The model under review builds one solid part; all positions refer to its coordinate system, in mm. A direction names the side the tool comes from. Round coordinates to 2 decimals unless told otherwise and drop trailing zeros. Order: outer loops, then holes, each group sorted by start corner. A loop starts at its lowest first (then second) coordinate and runs counter-clockwise, first axis right, second up.
1) Consider section B-B (z = -4.25). Give the boundary of the cut face in (x, y).
2) Consider section D-D (z = -24.5). Give the boundary of the cut face in (x, y).
3) Mouldability with a two-part tool opening along Z and no side actions: class faces 1 (the face through (2.521, -26.767, -5.591)), 2 (the face through (-2, -20, -8.5)), 3 (the face through (2, 0, -14)) as pulls with the +Z half, pulls with the -Z half, needs draft (parallel to the pull), parting line crosses it, or undercut.
4) Machinability: for faces 4 (the face through (1, -8, -4)), 5 (the face through (0, -20, 7)), 6 (the face through (8, -20, -44.5)), which of the approach directions +Z, -Z, +X, -X, +Y, -Y give a long, thin tool a straight path to every point of the face, cutting with its end or side? Answer none if there is none.
5) Clearance check with flat-ended pins moving along their axes: P1, Ø4, axis at y = -26.5, z = 4.5, coming from the -X side; P2, Ø11, axis at y = -30, z = -4.25, coming from the +X side; P3, Ø2, axis at y = -11, z = -5, coming from the +X side. State where each tip first meets the part, or that it passes through.
6) To check wall thickness, follow L1, parallel to Y at x = -2.55, z = -4.25; L2, parallel to Z at x = 2.7, y = -10; L3, parallel to Z at x = -0.85, y = -30. State the ranges of each line that lie inside material, in increasing order.
7) Consider section A-A (x = 6.5). Give the boundary of the cut face in (y, z), then the cut area to 3 significant figures.
from build123d import *

# Parameters (mm, degrees)
F1_DEPTH = 40
F2_R     = 1.5
F3_DEPTH = 25
F5_R     = 1
F4_R     = 3.5
F4_R_2   = 1.5
F6_DEPTH = 3
F7_R     = 0.99999


# Not quite as in the source:
# - a fillet or chamfer is up to 0.001 mm smaller than in the source, because OpenCascade refuses the exact size


with BuildPart() as f1:
    # F0 (on Front) → F1 (new body)
    with BuildSketch(Plane.XZ):
        Polygon((13, 15), (0, 15), (0, 0), (-5, 0), (-5, -8.5), (0, -8.5), (0, -48.5), (13, -48.5), (13, -42.5), (11, -42.5), (11, -44.5), (4, -44.5), (4, 11), (11, 11), (11, 9), (13, 9), align=None)
    extrude(amount=F1_DEPTH)

    # F2 (on face) → F3 (cut)
    with BuildSketch(Plane(origin=(-5, 0, 0), x_dir=(0, -1, 0), z_dir=(-1, 0, 0))):
        with Locations((10, -4.25)):
            Circle(F2_R)
        with Locations((30, -4.25)):
            Circle(F2_R)
    extrude(amount=-F3_DEPTH, mode=Mode.SUBTRACT)

    # F5
    f5_edges = [f1.edges().sort_by_distance(p)[0] for p in [
        (-5, -20, 0),
        (-5, -20, -8.5),
    ]]
    fillet(f5_edges, radius=F5_R)

    # F4 (on face) → F6 (cut)
    with BuildSketch(Plane.YZ.offset(4)):
        with Locations((-10, -4.25)):
            Circle(F4_R)
        with Locations((-10, -4.25)):
            Circle(F4_R_2, mode=Mode.SUBTRACT)
        with Locations((-30, -4.25)):
            Circle(F4_R)
        with Locations((-30, -4.25)):
            Circle(F4_R_2, mode=Mode.SUBTRACT)
    extrude(amount=-F6_DEPTH, mode=Mode.SUBTRACT)

    # F7 (radius 1 in the source; OpenCascade refuses exactly that, so slightly less here)
    f7_edges = [f1.edges().sort_by_distance(p)[0] for p in [
        (13, -20, 9),
        (11, -20, 9),
        (13, -20, 15),
        (0, -20, 15),
        (4, -20, 11),
        (0, -20, -48.5),
        (13, -20, -48.5),
        (13, -20, -42.5),
        (4, -20, -44.5),
        (11, -20, -42.5),
        (11, -20, -44.5),
        (11, -20, 11),
    ]]
    fillet(f7_edges, radius=F7_R)


solid = f1.part
Answer below:
1. outline: (-5, -40) - (4, -40) - (4, -33.5) - (1, -33.5) - (1, -31.5) - (-5, -31.5) - close; (-5, -28.5) - (1, -28.5) - (1, -26.5) - (4, -26.5) - (4, -13.5) - (1, -13.5) - (1, -11.5) - (-5, -11.5) - close; (-5, -8.5) - (1, -8.5) - (1, -6.5) - (4, -6.5) - (4, 0) - (-5, 0) - close
2. outline: (0, -40) - (4, -40) - (4, 0) - (0, 0) - close
3. face 1: undercut
3. face 2: pulls with the -Z half
3. face 3: needs draft
4. face 4: +X
4. face 5: +Z, -X, +Y, -Y
4. face 6: +Y, -Y
5. P1: stops at x = 0
5. P2: stops at x = 4
5. P3: stops at x = 1
6. L1: y = -40 to -31.5, -28.5 to -11.5, -8.5 to 0
6. L2: z = -48.5 to -7.75, -0.75 to 15
6. L3: z = -8.5 to -5.75, -2.75 to 0
7. outline: (-40, -48.5) - (0, -48.5) - (0, -44.5) - (-40, -44.5) - close; (-40, 11) - (0, 11) - (0, 15) - (-40, 15) - close
7. area: 320 mm2
